Work out the finished part from the listing and answer in its coordinate system (mm). Face numbers are marked on the shaded views. A direction names the side the tool comes from. Give positions to 0.01 mm unless a question says otherwise; leave off trailing zeros. Order: outer loops, then holes, each group sorted by start corner. A loop starts at its lowest first (then second) coordinate and runs counter-clockwise, first axis right, second up. Notation, with made-up numbers: (75, 66.5) - (103, 66.5) arc R30 ccw to (103, 89.5) - close; hole circle Ø8 at (-21, -5). An arc over 180 degrees is marked (long way). Put each result on its own line as item: value.
```python
from build123d import *

# Parameters (mm, degrees)
SKETCH1_W               = 54
SKETCH1_H               = 35
BOSS_EXTRUDE1_DEPTH     = 10
SKETCH2_W               = 22
SKETCH2_H               = 10
CUT_EXTRUDE1_DEPTH      = 29
SKETCH3_W               = 22
SKETCH3_H               = 10
CUT_EXTRUDE2_DEPTH      = 15
SKETCH5_R               = 1.6
CUT_EXTRUDE4_DEPTH      = 66.122960621
FILLET1_R               = 3
FILLET2_R               = 3
SKETCH8_W               = 10
SKETCH8_H               = 10
BOSS_EXTRUDE2_DEPTH     = 3
CUT_EXTRUDE5_DEPTH      = 4
CUT_EXTRUDE5_DEPTH_BACK = 15
SKETCH6_R               = 1.45
FILLET3_R               = 4


with BuildPart() as part:
    # Sketch1 → Boss-Extrude1 (new body)
    with BuildSketch(Plane(origin=(0, 0, 0), x_dir=(1, 0, 0), z_dir=(0, 1, 0))):
        with Locations((27, -17.5)):
            Rectangle(SKETCH1_W, SKETCH1_H)
    extrude(amount=BOSS_EXTRUDE1_DEPTH)

    # Sketch2 → Cut-Extrude1 (cut)
    with BuildSketch(Plane(origin=(54, 0, 0), x_dir=(0, 0, -1), z_dir=(1, 0, 0))):
        with Locations((-17.5, 5)):
            Rectangle(SKETCH2_W, SKETCH2_H)
    extrude(amount=-CUT_EXTRUDE1_DEPTH, mode=Mode.SUBTRACT)

    # Sketch3 → Cut-Extrude2 (cut)
    with BuildSketch(Plane.ZY):
        with Locations((17.5, 5)):
            Rectangle(SKETCH3_W, SKETCH3_H)
    extrude(amount=-CUT_EXTRUDE2_DEPTH, mode=Mode.SUBTRACT)

    # Sketch5 → Cut-Extrude4 (cut, through all)
    with BuildSketch(Plane.XY.offset(35)):
        with Locations((5, 5)):
            Circle(SKETCH5_R)
        with Locations((49, 5)):
            Circle(SKETCH5_R)
    extrude(amount=-CUT_EXTRUDE4_DEPTH, mode=Mode.SUBTRACT)

    # Fillet1
    fillet1_edges = [part.edges().sort_by_distance(p)[0] for p in [
        (54, 10, 31.75),
        (54, 0, 3.25),
        (54, 10, 3.25),
        (0, 0, 31.75),
        (0, 10, 31.75),
        (0, 10, 3.25),
        (54, 0, 31.75),
        (0, 0, 3.25),
    ]]
    fillet(fillet1_edges, radius=FILLET1_R)

    # Fillet2
    fillet2_edges = [part.edges().sort_by_distance(p)[0] for p in [
        (25, 5, 28.5),
        (25, 5, 6.5),
        (15, 5, 6.5),
        (15, 5, 28.5),
    ]]
    fillet(fillet2_edges, radius=FILLET2_R)

    # Sketch8 → Boss-Extrude2 (add)
    with BuildSketch(Plane.XY.offset(35)):
        with Locations((20, 5)):
            Rectangle(SKETCH8_W, SKETCH8_H)
    extrude(amount=BOSS_EXTRUDE2_DEPTH)

    # Sketch6 → Cut-Extrude5 (cut, two sides: drawn at the far end of the back side and taken through both)
    with BuildSketch(Plane.XY.offset(35).offset(-CUT_EXTRUDE5_DEPTH_BACK)):
        with Locations((19.5, 5)):
            Circle(SKETCH6_R)
    extrude(amount=CUT_EXTRUDE5_DEPTH + CUT_EXTRUDE5_DEPTH_BACK, mode=Mode.SUBTRACT)

    # Fillet3
    # the kernel refuses this fillet: 4 mm, written as the material it adds along each edge
    with BuildSketch(Plane(origin=(25, 10, 35), x_dir=(0, 0, 1), z_dir=(0, -1, 0))) as fillet3_piece_1:
        with BuildLine():
            CenterArc((4, -3.872983346), FILLET3_R, 104.477512186, 75.522487814)
            Line((0, -3.872983346), (-0.08, -3.872983346))
            Line((-0.08, -3.872983346), (-0.08, 0))
            Line((-0.08, 0), (0, 0.08))
            ThreePointArc((0, 0.08), (1.5, 0.08), (2.98, 0.077459667))
            Line((2.98, 0.077459667), (3, 0))
        make_face()
    extrude(amount=10)
    with BuildSketch(Plane(origin=(15, 0, 35), x_dir=(-1, 0, 0), z_dir=(0, 1, 0))) as fillet3_piece_2:
        with BuildLine():
            CenterArc((3.872983346, 4), FILLET3_R, 194.477512186, 75.522487814)
            Line((0, 3), (-0.077459667, 2.98))
            ThreePointArc((-0.077459667, 2.98), (-0.08, 1.5), (-0.08, 0))
            Line((-0.08, 0), (0, -0.08))
            Line((0, -0.08), (3.872983346, -0.08))
            Line((3.872983346, -0.08), (3.872983346, 0))
        make_face()
    extrude(amount=10)


solid = part.part
```
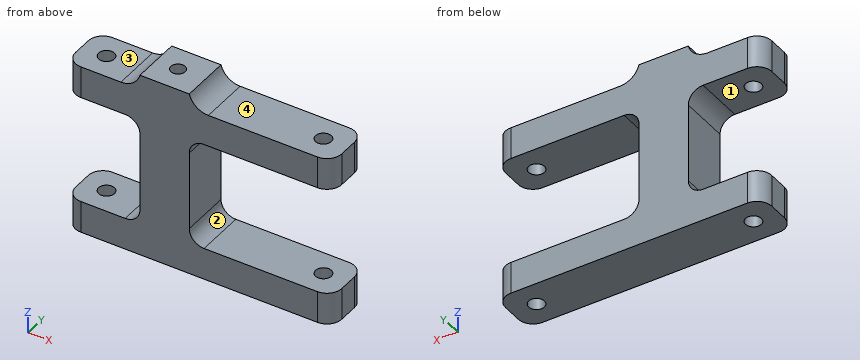
(1) Section C-C, the plane z = 5.5 is taken. Write down the section's boundary in (x, y).
Geometry check:
outline: (0, 3) arc R3 ccw to (3, 0) - (51, 0) arc R3 ccw to (54, 3) - (54, 7) arc R3 ccw to (51, 10) - (3, 10) arc R3 ccw to (0, 7) - close; hole circle Ø3.2 at (5, 5); hole circle Ø3.2 at (49, 5)
(2) Section B-B, the plane x = 49 is taken. Write down the section's boundary in (y, z), then the cut area to 3 significant figures.
Geometry check:
outline: (0, 0) - (3.4, 0) - (3.4, 6.5) - (0, 6.5) - close; (0, 28.5) - (3.4, 28.5) - (3.4, 35) - (0, 35) - close; (6.6, 0) - (10, 0) - (10, 6.5) - (6.6, 6.5) - close; (6.6, 28.5) - (10, 28.5) - (10, 35) - (6.6, 35) - close
area: 88.4 mm²
(3) Given pin 1 (0.9 mm diameter, centred on x = 19.5, y = 4.5, fed in from +Z); pin 2 (2 mm diameter, centred on y = 1.5, z = 23, fed in from +X); pin 3 (1.5 mm diameter, centred on x = 46.5, y = 9, fed in from +Z); pin 4 (3.5 mm diameter, centred on x = 5, y = 5, fed in from -Z), each flat-ended and moving along its own axis, determine where each tip first touches the part or whether it passes through.
Geometry check:
pin 1: stops at z = 20
pin 2: stops at x = 25
pin 3: stops at z = 35
pin 4: stops at z = 0
(4) Section A-A, the plane x = 29.5 is taken. Write down the section's boundary in (y, z), then the cut area to 3 significant figures.
Geometry check:
outline: (0, 0) - (10, 0) - (10, 6.5) - (0, 6.5) - close; (0, 28.5) - (10, 28.5) - (10, 35) - (0, 35) - close
area: 130 mm²
(5) Straight lines are drawn through the part: line 1 (Z direction, x = 7, y = 8); line 2 (X direction, y = 4.25, z = 31.5); line 3 (Y direction, x = 5, z = 30). For each, find the intervals that lie inside material, in ascending order.
Geometry check:
line 1: z = 0 to 6.5, 28.5 to 35
line 2: x = 0 to 3.59, 6.41 to 18.26, 20.74 to 47.59, 50.41 to 54
line 3: y = 0 to 3.4, 6.6 to 10
(6) A tool of negligible diameter and unlimited length cuts with its end or side. For the marked faces 1, 2, 3 and 4, from which of +Z, -Z, +X, -X, +Y, -Y can it reach the whole face along a straight path? Write none if from no direction.
Geometry check:
face 1: -X, +Y, -Y
face 2: +X, +Y, -Y
face 3: +Z, -X, +Y, -Y
face 4: +Z, +X, +Y, -Y
(7) Section D-D, the plane y = 5 is taken. Count the separate pieces of the cut face and the enclosed holes in it, then the cut area to 3 significant figures.
Geometry check:
separate pieces: 5
enclosed holes: 0
area: 830 mm²
